Verification items for the finished model (mm, model axes). Face numbers are marked on the shaded views. A direction names the side the tool comes from. Give positions to 0.01 mm unless a question says otherwise; leave off trailing zeros. Loops run counter-clockwise (first coordinate to the right, second up) from the corner with the lowest first, then second, coordinate; pieces in that order, holes last. Notation, with made-up numbers: M 13,-11 L 58,-11 A16 ccw 58,1 Z; hole C 35.5,-26.5 d8. An arc over 180 degrees is marked long. Use a Markdown table: item, result.
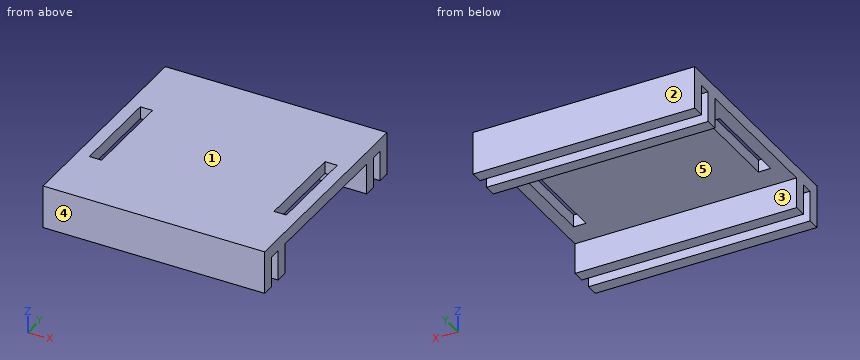
from build123d import *

# Parameters (mm, degrees)
F0_W     = 36
F0_H     = 36
F0_W_2   = 2
F0_H_2   = 15
F1_DEPTH = 2
F2_W     = 36
F2_H     = 2
F3_DEPTH = 5


with BuildPart() as f1:
    # F0 (on Top) → F1 (new body)
    with BuildSketch(Plane.XY):
        with Locations((1.428571, 2.255185)):
            Rectangle(F0_W, F0_H)
        with Locations((-13.571429, 1.755185)):
            Rectangle(F0_W_2, F0_H_2, mode=Mode.SUBTRACT)
        with Locations((16.428571, 1.755185)):
            Rectangle(F0_W_2, F0_H_2, mode=Mode.SUBTRACT)
    extrude(amount=F1_DEPTH)

    # F2 (on face) → F3 (join)
    with BuildSketch(Plane(origin=(0, 0, 0), x_dir=(1, 0, 0), z_dir=(0, 0, -1))):
        with Locations((1.428571, 14.744815)):
            Rectangle(F2_W, F2_H)
        with Locations((1.428571, 10.744815)):
            Rectangle(F2_W, F2_H)
        with Locations((1.428571, -19.255185)):
            Rectangle(F2_W, F2_H)
        with Locations((1.428571, -15.255185)):
            Rectangle(F2_W, F2_H)
    extrude(amount=F3_DEPTH)


solid = f1.part
(1) Cross-section at C-C on z = 0.75. Record the cut outline in (x, y), then the cut area to 3 significant figures.
Results below:
| item | result |
|---|---|
| outline | M -16.57,-15.74 L 19.43,-15.74 L 19.43,20.26 L -16.57,20.26 Z; hole M -14.57,-5.74 L -12.57,-5.74 L -12.57,9.26 L -14.57,9.26 Z; hole M 15.43,-5.74 L 17.43,-5.74 L 17.43,9.26 L 15.43,9.26 Z |
| area | 1,240 mm^2 |
(2) Cross-section at A-A on y = 5. Record the cut outline in (x, z), then the cut area to 3 significant figures.
Results below:
| item | result |
|---|---|
| outline | M -16.57,0 L -14.57,0 L -14.57,2 L -16.57,2 Z; M -12.57,0 L 15.43,0 L 15.43,2 L -12.57,2 Z; M 17.43,0 L 19.43,0 L 19.43,2 L 17.43,2 Z |
| area | 64.0 mm^2 |
(3) Draft check along Y on the marked faces 1, 2 and 3. Enter one of: +Y half, -Y half, draft (parallel to the pull), parting line (faces both ways), or undercut.
Results below:
| item | result |
|---|---|
| face 1 | draft |
| face 2 | +Y half |
| face 3 | undercut |
(4) Gauge pin test, flat end, axial feed: P1, Ø4, axis at x = 12.5, y = -5.5, coming from the -Z side. Record the tip position at first contact, or that the pin passes through.
Results below:
| item | result |
|---|---|
| P1 | z = 0 |
(5) Set-up check for the marked faces 4 and 5: record each of +Z, -Z, +X, -X, +Y, -Y from which the full face is reachable in a straight line by a thin tool's end or side.
Results below:
| item | result |
|---|---|
| face 4 | +Z, -Z, +X, -X, -Y |
| face 5 | -Z, +X, -X |
(6) Cross-section at B-B on x = 16.5. Record the cut outline in (y, z).
Results below:
| item | result |
|---|---|
| outline | M -15.74,-5 L -13.74,-5 L -13.74,0 L -11.74,0 L -11.74,-5 L -9.74,-5 L -9.74,0 L -5.74,0 L -5.74,2 L -15.74,2 Z; M 9.26,0 L 14.26,0 L 14.26,-5 L 16.26,-5 L 16.26,0 L 18.26,0 L 18.26,-5 L 20.26,-5 L 20.26,2 L 9.26,2 Z |
(7) Cross-section at D-D on z = -3.5. Record the cut outline in (x, y), then the cut area to 3 significant figures.
Results below:
| item | result |
|---|---|
| outline | M -16.57,-15.74 L 19.43,-15.74 L 19.43,-13.74 L -16.57,-13.74 Z; M -16.57,-11.74 L 19.43,-11.74 L 19.43,-9.74 L -16.57,-9.74 Z; M -16.57,14.26 L 19.43,14.26 L 19.43,16.26 L -16.57,16.26 Z; M -16.57,18.26 L 19.43,18.26 L 19.43,20.26 L -16.57,20.26 Z |
| area | 288 mm^2 |
(8) Material ranges on line 1 (Y direction, x = 17.5, z = -4.5); line 2 (Y direction, x = 16, z = 0.75); line 3 (Z direction, x = 13, y = 2), recorded low to high.
Results below:
| item | result |
|---|---|
| line 1 | -15.74 to -13.74, -11.74 to -9.74, 14.26 to 16.26, 18.26 to 20.26 |
| line 2 | -15.74 to -5.74, 9.26 to 20.26 |
| line 3 | 0 to 2 |
